Geometry: final body of the model. Coordinates: model frame, mm. A direction names the side the tool comes from. Give positions to 0.01 mm unless a question says otherwise; leave off trailing zeros. Write each loop counter-clockwise with the first axis right and the second up, starting at its lowest first coordinate (ties: lowest second). Pieces come first, ordered by that corner, then holes. Notation, with made-up numbers: M -5,23 L 18,23 A23 cw 18,35 Z; hole C -35,14.25 d8. An arc over 180 degrees is marked long. Use one line per item in the form item = value. Start each with the question number.
Item 1: Contact query for flat-ended pins moving along their axis: P1, Ø2, axis at y = 208, z = -8, coming from the -X side; P2, Ø6, axis at y = 346, z = -5, coming from the +X side; P3, Ø2, axis at x = 3.5, y = 885, coming from the -Z side. Output: stop coordinate, or through.
Item 2: Section query C-C on y = 386. Return loops of the section in (x, z), then the cut area to 3 significant figures.
Item 3: Section query A-A on z = 8. Return loops of the section in (x, y).
Item 4: Material intervals for line 1 along X through (y, z) = (946, -0.5); line 2 along Z through (x, y) = (1.75, 215); line 3 along X through (y, z) = (112, -2.5), sorted ascending. Write a range as from..to.
Item 5: Section query B-B on x = 5. Return loops of the section in (y, z).
Item 6: Access query for faces 1 (the cylindrical face through (-7.7, 626.1, -10.1)), 2 (the flat face through (0, -25.4, 0)). Directions: +Z, -Z, +X, -X, +Y, -Y. A direction counts if a zero-diameter tool reaches every point of the face in a straight line with its end or side. Return the directions, or none.
from build123d import *

# Parameters (mm, degrees)
SKETCH1_R           = 12.7
BOSS_EXTRUDE1_DEPTH = 25.4
SKETCH1_3_R         = 12.7
BOSS_EXTRUDE2_DEPTH = 1270


with BuildPart() as part:
    # Sketch1 → Boss-Extrude1 (new body)
    with BuildSketch(Plane(origin=(0, 0, 0), x_dir=(1, 0, 0), z_dir=(0, 1, 0))):
        with BuildLine():
            Line((0, 12.7), (-12.7, 12.7))
            Line((-12.7, 12.7), (-12.7, -3e-08))
            ThreePointArc((-12.7, -3e-08), (-8.980256132, 8.98025611), (0, 12.7))
        make_face()
        with BuildLine():
            ThreePointArc((0, -12.7), (-8.98025611, -8.980256132), (-12.7, -3e-08))
            Line((-12.7, -3e-08), (-12.7, -12.7))
            Line((-12.7, -12.7), (0, -12.7))
        make_face()
        Circle(SKETCH1_R)
        with BuildLine():
            Line((12.7, 12.7), (0, 12.7))
            ThreePointArc((0, 12.7), (8.980256121, 8.980256121), (12.7, 0))
            Line((12.7, 0), (12.7, 12.7))
        make_face()
        with BuildLine():
            Line((12.7, -12.7), (12.7, 0))
            ThreePointArc((12.7, 0), (8.980256121, -8.980256121), (0, -12.7))
            Line((0, -12.7), (12.7, -12.7))
        make_face()
    extrude(amount=-BOSS_EXTRUDE1_DEPTH)

    # Sketch1_3 → Boss-Extrude2 (add)
    with BuildSketch(Plane(origin=(0, 0, 0), x_dir=(1, 0, 0), z_dir=(0, 1, 0))):
        with Locations(Location((0, 0, 0), (0, 0, 270))):
            Circle(SKETCH1_3_R)
    extrude(amount=BOSS_EXTRUDE2_DEPTH)


solid = part.part
Answer sheet:
q1.P1 = -10.6
q1.P2 = 12.54
q1.P3 = -12.45
q2.outline = C 0,0 d25.4
q2.area = 507 mm2
q3.outline = M -12.7,-25.4 L 12.7,-25.4 L 12.7,0 L 9.86,0 L 9.86,1270 L -9.86,1270 L -9.86,0 L -12.7,0 Z
q4.line_1 = -12.69..12.69
q4.line_2 = -12.58..12.58
q4.line_3 = -12.45..12.45
q5.outline = M -25.4,-12.7 L 0,-12.7 L 0,-11.67 L 1270,-11.67 L 1270,11.67 L 0,11.67 L 0,12.7 L -25.4,12.7 Z
q6.face_1 = +Y
q6.face_2 = +Z, -Z, +X, -X, -Y
